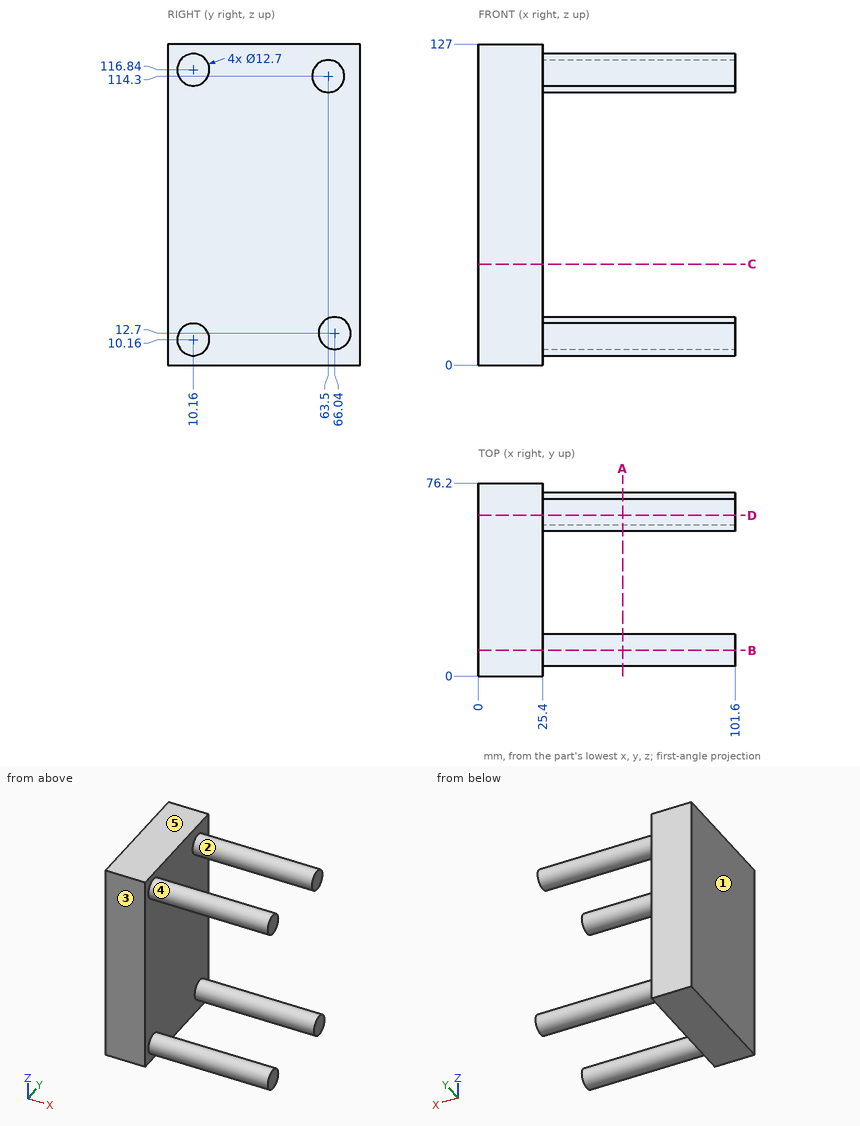
Study the drawing (mm; zero at the part's minimum x, y, z) and answer. A direction names the side the tool comes from. Coordinates: 2 decimals unless noted, no trailing zeros. Order: outer loops, then holes, each group sorted by start corner. A loop starts at its lowest first (then second) coordinate and runs counter-clockwise, first axis right, second up. Notation, with made-up numbers: M 11,-10 L 70,-10 A26 cw 70,9 Z; hole C 47,18 d3. An arc over 180 degrees is marked long. Answer as a JSON object with one key per item and string values. Group by question number.
1. Determine the mould class of the marked faces 1, 2 and 3 for opening direction Y: released by +Y, released by -Y, zero draft, split by the parting line, or undercut.
2. Section D-D on y = 63.5 is taken. Write down the section's boundary in (x, z), then the cut area to 3 significant figures.
3. Section C-C on z = 40 is taken. Write down the section's boundary in (x, y), then the cut area to 3 significant figures.
4. Flat-ended cylindrical pins translate along their axes: P1, Ø2, axis at y = 63.5, z = 90.5, coming from the -X side; P2, Ø1.5, axis at x = 36, y = 61.5, coming from the -Z side; P3, Ø3, axis at x = 84.5, y = 8, coming from the +Z side; P4, Ø10, axis at x = 47.5, z = 104, coming from the +Y side. Find the tip coordinate at first contact, or state that the pin passes through.
5. Section B-B on y = 10.16 is taken. Write down the section's boundary in (x, z).
6. A tool of negligible diameter and unlimited length cuts with its end or side. For the marked faces 4 and 5, from which of +Z, -Z, +X, -X, +Y, -Y can it reach the whole face along a straight path? Write none if from no direction.
7. Straight lines are drawn through the part: line 1 (X direction, y = 39.5, z = 78.5); line 2 (Y direction, x = 37.5, z = 116); line 3 (Y direction, x = 46, z = 114). For each, find the intervals that lie inside material, in ascending order.
8. Section A-A on x = 57 is taken. Write down the section's boundary in (y, z), then the cut area to 3 significant figures.
Values follow:
{
 "1": {"face 1": "zero draft", "face 2": "undercut", "face 3": "released by -Y"},
 "2": {"outline": "M 0,0 L 25.4,0 L 25.4,6.88 L 101.6,6.88 L 101.6,18.52 L 25.4,18.52 L 25.4,107.95 L 101.6,107.95 L 101.6,120.65 L 25.4,120.65 L 25.4,127 L 0,127 Z", "area": "5,080 mm2"},
 "3": {"outline": "M 0,0 L 25.4,0 L 25.4,76.2 L 0,76.2 Z", "area": "1,940 mm2"},
 "4": {"P1": "x = 0", "P2": "z = 7.61", "P3": "z = 123.16", "P4": "y = 67"},
 "5": {"outline": "M 0,0 L 25.4,0 L 25.4,3.81 L 101.6,3.81 L 101.6,16.51 L 25.4,16.51 L 25.4,110.49 L 101.6,110.49 L 101.6,123.19 L 25.4,123.19 L 25.4,127 L 0,127 Z"},
 "6": {"face 4": "+X", "face 5": "+Z, +X, -X, +Y, -Y"},
 "7": {"line 1": "0 to 25.4", "line 2": "3.87 to 16.45, 57.38 to 69.62", "line 3": "4.48 to 15.84, 57.16 to 69.84"},
 "8": {"outline": "C 10.16,10.16 d12.7; C 10.16,116.84 d12.7; C 63.5,114.3 d12.7; C 66.04,12.7 d12.7", "area": "507 mm2"}
}
